The listing builds one solid part. Answer for the finished solid, in the listing's coordinates (mm). Round coordinates to 2 decimals unless told otherwise and drop trailing zeros. Write each loop counter-clockwise with the first axis right and the second up, starting at its lowest first coordinate (ties: lowest second). Pieces come first, ordered by that corner, then holes. Notation, with made-up numbers: (19.25, 62) - (29.25, 62) arc R9 ccw to (29.25, 79) - close; hole circle Ø9 at (29, -25.5). An arc over 180 degrees is marked (long way). Use a Markdown table: item, result. Add a question column.
1) A cutting plane is placed at C-C (x = 1.5). Give the vertices of the cut face in (y, z).
2) A cutting plane is placed at A-A (y = 0). Give the vertices of the cut face in (x, z), then the cut area to 3 significant figures.
3) A cutting plane is placed at B-B (z = 76.2). Give the vertices of the cut face in (x, y), then the cut area to 3 significant figures.
4) Determine the mould class of faces 1 (the flat face through (-38.1, 0, 63)), 2 (the cylindrical face through (-0.53, 1.38, 108.1)), 3 (the flat face through (-1, 25.4, 63)) for opening direction Y: +Y half, -Y half, draft (parallel to the pull), parting line (faces both ways), or undercut.
5) A cutting plane is placed at D-D (z = 114.3). Give the vertices of the cut face in (x, y), then the cut area to 3 significant figures.
6) Find the intervals of material crossed by probe 1 along Z at (x, y) = (-10, 0); probe 2 along Y at (x, z) = (-9, 76); probe 3 along Z at (x, y) = (22, -3), in increasing order. Write a range as from..to.
```python
from build123d import *

# Parameters (mm, degrees)
F0_W     = 76.2
F0_H     = 50.8
F1_DEPTH = 127
F3_D     = 25.4
F5_D     = 12.7


with BuildPart() as f1:
    # F0 (on Top) → F1 (new body)
    with BuildSketch(Plane.XY):
        Rectangle(F0_W, F0_H)
    extrude(amount=F1_DEPTH)

    # F3 (through all)
    with Locations(Plane.YZ.offset(38.1)):
        with Locations((0, 76.2)):
            Hole(F3_D / 2)

    # F5 (through all)
    with Locations(Plane.YZ.offset(38.1)):
        with Locations((0, 114.3)):
            Hole(F5_D / 2)


solid = f1.part
```
Entries:
| question | item | result |
|---|---|---|
| 1 | outline | (-25.4, 0) - (25.4, 0) - (25.4, 127) - (-25.4, 127) - close; hole circle Ø25.4 at (0, 76.2); hole circle Ø12.7 at (0, 114.3) |
| 2 | outline | (-38.1, 0) - (38.1, 0) - (38.1, 63.5) - (-38.1, 63.5) - close; (-38.1, 88.9) - (38.1, 88.9) - (38.1, 107.95) - (-38.1, 107.95) - close; (-38.1, 120.65) - (38.1, 120.65) - (38.1, 127) - (-38.1, 127) - close |
| 2 | area | 6,770 mm² |
| 3 | outline | (-38.1, -25.4) - (38.1, -25.4) - (38.1, -12.7) - (-38.1, -12.7) - close; (-38.1, 12.7) - (38.1, 12.7) - (38.1, 25.4) - (-38.1, 25.4) - close |
| 3 | area | 1,940 mm² |
| 4 | face 1 | draft |
| 4 | face 2 | undercut |
| 4 | face 3 | +Y half |
| 5 | outline | (-38.1, -25.4) - (38.1, -25.4) - (38.1, -6.35) - (-38.1, -6.35) - close; (-38.1, 6.35) - (38.1, 6.35) - (38.1, 25.4) - (-38.1, 25.4) - close |
| 5 | area | 2,900 mm² |
| 6 | probe 1 | z = 0..63.5, 88.9..107.95, 120.65..127 |
| 6 | probe 2 | y = -25.4..-12.7, 12.7..25.4 |
| 6 | probe 3 | z = 0..63.86, 88.54..108.7, 119.9..127 |
